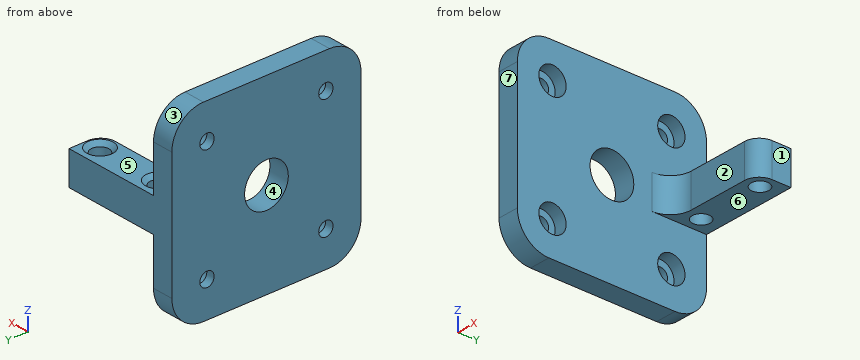
```python
from build123d import *

# Parameters (mm, degrees)
SKETCH1_R                      = 5.205
SKETCH1_W                      = 8
SKETCH1_H                      = 8
BOSS_EXTRUDE1_DEPTH            = 5
SKETCH1_3_W                    = 8
SKETCH1_3_H                    = 8
BOSS_EXTRUDE2_DEPTH            = 28
FILLET1_R                      = 7.5
FILLET2_R                      = 5
FILLET3_R                      = 3.5
SKETCH2_R                      = 2.125
CUT_EXTRUDE1_DEPTH             = 23.5
CUT_EXTRUDE1_DEPTH_BACK        = 23.5
CBORE_FOR_M3_SHCS1_D           = 3.4
CBORE_FOR_M3_SHCS1_CBORE_D     = 6.5
CBORE_FOR_M3_SHCS1_CBORE_DEPTH = 3
CHAMFER1_SIZE                  = 1


with BuildPart() as part:
    # Sketch1 → Boss-Extrude1 (new body)
    with BuildSketch(Plane(origin=(0, 0, 0), x_dir=(0, 0, -1), z_dir=(1, 0, 0))):
        Polygon((-22.5, 22.5), (-22.5, -22.5), (22.5, -22.5), (22.5, 22.5), (4, 22.5), (4, 14.5), (-4, 14.5), (-4, 22.5), align=None)
        Circle(SKETCH1_R, mode=Mode.SUBTRACT)
        with Locations((0, 18.5)):
            Rectangle(SKETCH1_W, SKETCH1_H)
    extrude(amount=BOSS_EXTRUDE1_DEPTH)

    # Sketch1<3> → Boss-Extrude2 (add)
    with BuildSketch(Plane(origin=(0, 0, 0), x_dir=(0, 0, -1), z_dir=(1, 0, 0))):
        with Locations((0, 18.5)):
            Rectangle(SKETCH1_3_W, SKETCH1_3_H)
    extrude(amount=BOSS_EXTRUDE2_DEPTH)

    # Fillet1
    fillet1_edges = [part.edges().sort_by_distance(p)[0] for p in [
        (2.5, 22.5, -22.5),
        (2.5, -22.5, -22.5),
        (2.5, -22.5, 22.5),
        (2.5, 22.5, 22.5),
    ]]
    fillet(fillet1_edges, radius=FILLET1_R)

    # Fillet2
    fillet2_edges = [part.edges().sort_by_distance(p)[0] for p in [
        (5, 14.5, 0),
    ]]
    fillet(fillet2_edges, radius=FILLET2_R)

    # Fillet3
    fillet3_edges = [part.edges().sort_by_distance(p)[0] for p in [
        (28, 14.5, 0),
    ]]
    fillet(fillet3_edges, radius=FILLET3_R)

    # Sketch2 → Cut-Extrude1 (cut, two sides)
    with BuildSketch(Plane.XY) as cut_extrude1_sk:
        with Locations((8.6, 18.1)):
            Circle(SKETCH2_R)
        with Locations((24.6, 18.1)):
            Circle(SKETCH2_R)
    extrude(amount=CUT_EXTRUDE1_DEPTH, mode=Mode.SUBTRACT)
    extrude(cut_extrude1_sk.sketch, amount=-CUT_EXTRUDE1_DEPTH_BACK, mode=Mode.SUBTRACT)

    # CBORE for M3 SHCS1 (through all)
    with Locations(Plane(origin=(5, 0, 0), x_dir=(0, 0, -1), z_dir=(1, 0, 0))):
        with Locations((-14.142135624, 14.142135624), (14.142135624, 14.142135624), (-14.142135624, -14.142135624), (14.142135624, -14.142135624)):
            CounterBoreHole(CBORE_FOR_M3_SHCS1_D / 2, CBORE_FOR_M3_SHCS1_CBORE_D / 2, CBORE_FOR_M3_SHCS1_CBORE_DEPTH)

    # Chamfer1
    chamfer1_edges = [part.edges().sort_by_distance(p)[0] for p in [
        (6.475, 18.1, 4),
        (22.475, 18.1, 4),
    ]]
    chamfer(chamfer1_edges, length=CHAMFER1_SIZE)


solid = part.part
```
Build history of the part. All positions in model axes, mm. Face numbers are marked on the shaded views. A direction names the side the tool comes from. Give positions to 0.01 mm unless a question says otherwise; leave off trailing zeros. Order: outer loops, then holes, each group sorted by start corner. A loop starts at its lowest first (then second) coordinate and runs counter-clockwise, first axis right, second up. Notation, with made-up numbers: M -15,52.25 L 26,52.25 A15 cw 26,58.25 Z; hole C 45.5,54.25 d1. An arc over 180 degrees is marked long. Return JSON: item names as keys, results as strings.
Q1. Band-saw the part on A-A (x = 8.6). Give the cut face in (y, z) (3 decimals), then the cut area to 3 significant figures.
Answer list:
{"outline": "M 14.3,-4 L 15.975,-4 L 15.975,3 L 14.975,4 L 14.3,4 Z; M 20.225,-4 L 22.5,-4 L 22.5,4 L 21.225,4 L 20.225,3 Z", "area": "30.6 mm^2"}
Q2. Band-saw the part on B-B (y = 0). Give the cut face in (x, z) (3 decimals), then the cut area to 3 significant figures.
Answer list:
{"outline": "M 0,-22.5 L 5,-22.5 L 5,-5.205 L 0,-5.205 Z; M 0,5.205 L 5,5.205 L 5,22.5 L 0,22.5 Z", "area": "173 mm^2"}
Q3. Band-saw the part on D-D (y = -4.5). Give the cut face in (x, z).
Answer list:
{"outline": "M 0,-22.5 L 5,-22.5 L 5,-2.62 L 0,-2.62 Z; M 0,2.62 L 5,2.62 L 5,22.5 L 0,22.5 Z"}
Q4. Wall check: probe 1 along Z at (x, y) = (3, -11.5); probe 2 along Y at (x, z) = (20, -1); probe 3 along X at (y, z) = (3.5, -20). Give the ranges that are in metal, low to high. Write a range as from..to.
Answer list:
{"probe 1": "z = -22.5..-16.03, -12.25..12.25, 16.03..22.5", "probe 2": "y = 14.5..22.5", "probe 3": "x = 0..5"}
Q5. Band-saw the part on C-C (x = 14.25). Give the cut face in (y, z), then the cut area to 3 significant figures.
Answer list:
{"outline": "M 14.5,-4 L 22.5,-4 L 22.5,4 L 14.5,4 Z", "area": "64.0 mm^2"}
Q6. 3-axis set-ups, long thin cutter, end or side, ignore diameter. For the marked faces 5, 6 and 7: which of +Z, -Z, +X, -X, +Y, -Y reach the whole face in a straight line?
Answer list:
{"face 5": "+Z, +X, +Y, -Y", "face 6": "-Z, +X, +Y, -Y", "face 7": "+Z, -Z, +X, -X, -Y"}
Q7. Two-plate mould, pull along Y, no slides. Class the marked faces 1, 2, 3 and 4: pulls with the +Y half, pulls with the -Y half, needs draft (parallel to the pull), parting line crosses it, or undercut.
Answer list:
{"face 1": "needs draft", "face 2": "pulls with the -Y half", "face 3": "pulls with the +Y half", "face 4": "undercut"}
Q8. Flat gauge pins, fed straight in: pin 1 (7 mm diameter, centred on y = -14.5, z = -15, fed in from +X); pin 2 (7 mm diameter, centred on x = 24.6, y = 18.1, fed in from -Z); pin 3 (5.5 mm diameter, centred on x = 24.6, y = 18.1, fed in from +Z) (3 decimals). Where does each tip first touch, or does it go through?
Answer list:
{"pin 1": "stops at x = 5", "pin 2": "stops at z = -4", "pin 3": "stops at z = 3.625"}
